Input: part model. Units: mm. Frame: model coordinates. Face numbers are marked on the shaded views. A direction names the side the tool comes from. Coordinates: 2 decimals unless noted, no trailing zeros. Loops run counter-clockwise (first coordinate to the right, second up) from the corner with the lowest first, then second, coordinate; pieces in that order, holes last. Notation, with made-up numbers: M 8,58 L 64,58 A22 ccw 64,79 Z; hole C 38.25,-17 d11. An arc over 180 degrees is marked long. Use a Markdown table: item, result. Add a question column.
1. Section D-D on y = 29. Output: boundary loops of the cut face in (x, z), then the cut area to 3 significant figures.
2. Section B-B on x = 30. Output: boundary loops of the cut face in (y, z), then the cut area to 3 significant figures.
3. Section C-C on z = 22.5. Output: boundary loops of the cut face in (x, y), then the cut area to 3 significant figures.
4. Set-up query: the marked faces 1, 2 and 3. Return all of +Z, -Z, +X, -X, +Y, -Y with unobstructed straight access to the full face (end or side cutting, diameter ignored); none if empty.
5. Draft query along Y for the marked faces 4, 5 and 6. Return one class per face: +Y half, -Y half, draft (parallel to the pull), parting line (faces both ways), or undercut.
6. Pin query (flat end, axial travel): pin 1 (10 mm diameter, centred on x = 31, y = 8, fed in from -Z); pin 2 (3.5 mm diameter, centred on y = 20, z = 27, fed in from -X); pin 3 (9.5 mm diameter, centred on x = 5.5, y = 27.5, fed in from +Z); pin 4 (19 mm diameter, centred on x = 33, y = 26, fed in from -Z). Return the tip coordinate at first contact, or that it passes through.
7. Section A-A on z = 10.5. Output: boundary loops of the cut face in (x, y).
8. Line query: L1, parallel to X at y = 24, z = 21.75; L2, parallel to X at y = 24, z = 27.75; L3, parallel to Y at x = 76, z = 4. Output: solid intervals per line, ascending. Write a range as [from, to].
```python
from build123d import *

# Parameters (mm, degrees)
SKETCH1_W           = 84
SKETCH1_H           = 48
SKETCH1_R           = 12
BOSS_EXTRUDE1_DEPTH = 36
SKETCH2_W           = 12
SKETCH2_H           = 12
CUT_EXTRUDE1_DEPTH  = 49
SKETCH3_W           = 12
SKETCH3_H           = 24
CUT_EXTRUDE2_DEPTH  = 85
SKETCH5_W           = 12
SKETCH5_H           = 12
CUT_EXTRUDE4_DEPTH  = 24


with BuildPart() as part:
    # Sketch1 → Boss-Extrude1 (new body)
    with BuildSketch(Plane.XY):
        with Locations((42, 24)):
            Rectangle(SKETCH1_W, SKETCH1_H)
        with BuildLine():
            Line((36, 24), (36, 12))
            Line((36, 12), (24, 12))
            Line((24, 12), (24, 24))
            ThreePointArc((24, 24), (30, 30.000000202), (36, 24))
        make_face(mode=Mode.SUBTRACT)
        with Locations((60, 24)):
            Circle(SKETCH1_R, mode=Mode.SUBTRACT)
    extrude(amount=BOSS_EXTRUDE1_DEPTH)

    # Sketch2 → Cut-Extrude1 (cut, through all)
    with BuildSketch(Plane(origin=(0, 48, 0), x_dir=(1, 0, 0), z_dir=(0, 1, 0))):
        with Locations((6, -30)):
            Rectangle(SKETCH2_W, SKETCH2_H)
    extrude(amount=-CUT_EXTRUDE1_DEPTH, mode=Mode.SUBTRACT)

    # Sketch3 → Cut-Extrude2 (cut, through all)
    with BuildSketch(Plane.ZY):
        with Locations((6, 24)):
            Rectangle(SKETCH3_W, SKETCH3_H)
    extrude(amount=-CUT_EXTRUDE2_DEPTH, mode=Mode.SUBTRACT)

    # Sketch5 → Cut-Extrude4 (cut)
    with BuildSketch(Plane.XY.offset(36)):
        with Locations((30, 6)):
            Rectangle(SKETCH5_W, SKETCH5_H)
    extrude(amount=-CUT_EXTRUDE4_DEPTH, mode=Mode.SUBTRACT)


solid = part.part
```
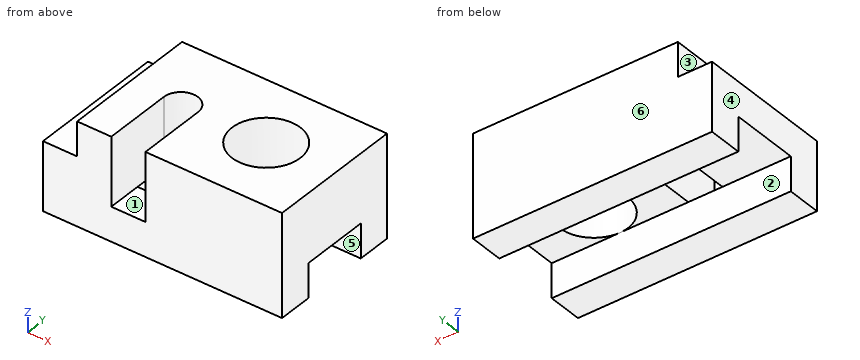
Answers below:
| question | item | result |
|---|---|---|
| 1 | outline | M 0,12 L 26.68,12 L 26.68,36 L 12,36 L 12,24 L 0,24 Z; M 33.32,12 L 49.09,12 L 49.09,36 L 33.32,36 Z; M 70.91,12 L 84,12 L 84,36 L 70.91,36 Z |
| 1 | area | 1,190 mm² |
| 2 | outline | M 0,0 L 12,0 L 12,12 L 0,12 Z; M 30,12 L 36,12 L 36,0 L 48,0 L 48,36 L 30,36 Z |
| 2 | area | 720 mm² |
| 3 | outline | M 0,0 L 24,0 L 24,24 A6 cw 36,24 L 36,0 L 84,0 L 84,48 L 0,48 Z; hole C 60,24 d24 |
| 3 | area | 3,240 mm² |
| 4 | face 1 | +Z, -Y |
| 4 | face 2 | -Z, +X, -X |
| 4 | face 3 | +Z, -X, +Y, -Y |
| 5 | face 4 | draft |
| 5 | face 5 | undercut |
| 5 | face 6 | +Y half |
| 6 | pin 1 | stops at z = 0 |
| 6 | pin 2 | stops at x = 12 |
| 6 | pin 3 | stops at z = 24 |
| 6 | pin 4 | stops at z = 12 |
| 7 | outline | M 0,0 L 84,0 L 84,12 L 0,12 Z; M 0,36 L 84,36 L 84,48 L 0,48 Z |
| 8 | L1 | x = [0, 24], [36, 48], [72, 84] |
| 8 | L2 | x = [12, 24], [36, 48], [72, 84] |
| 8 | L3 | y = [0, 12], [36, 48] |
